```python
from build123d import *

# Parameters (mm, degrees)
BOSS_EXTRUDE1_DEPTH = 1.5
CUT_EXTRUDE6_DEPTH  = 11.5
CUT_EXTRUDE7_DEPTH  = 11.5


with BuildPart() as part:
    # 3DSketch1 → Boss-Extrude1 (new, along a direction that is not the sketch's normal)
    with BuildSketch(Plane(origin=(-11.663984258, 358.235252064, 0), x_dir=(0.8242948566390451, -0.5203008813923206, 0.22321510285101764), z_dir=(-0.26553281531955075, -0.007074831163105001, 0.964075863587761))):
        Polygon((0, 0), (489.889504132, 504.199636792), (815.132069395, 0), (238.511214526, -369.746400314), align=None)
    extrude(amount=BOSS_EXTRUDE1_DEPTH, dir=(0, 0, 1))

    # Sketch2 → Cut-Extrude6 (cut)
    with BuildSketch(Plane(origin=(-0.533410404, -0.014212136, 1.936664949), x_dir=(0.9641018224173596, -0.0019485492019291684, 0.26552566574162595), z_dir=(-0.26553281531954953, -0.007074831163105186, 0.9640758635877613))):
        with BuildLine():
            ThreePointArc((635.382584147, -65.776722047), (337.840777347, 133.826895304), (50.610501363, -80.349432548))
            Line((50.610501363, -80.349432548), (635.382584147, -65.776722047))
        make_face()
    extrude(amount=-CUT_EXTRUDE6_DEPTH, mode=Mode.SUBTRACT)

    # Sketch3 → Cut-Extrude7 (cut)
    with BuildSketch(Plane(origin=(-0.533410404, -0.014212136, 1.936664949), x_dir=(0.9641018224173596, -0.0019485492019291684, 0.26552566574162595), z_dir=(-0.26553281531954953, -0.007074831163105186, 0.9640758635877613))):
        Polygon((50.610501363, -80.349432548), (50.610501363, -106.198699681), (633.779172918, -106.198699681), (635.382584147, -65.776722047), (592.923417402, -33.337692785), (162.965228398, -33.337692785), align=None)
    extrude(amount=-CUT_EXTRUDE7_DEPTH, mode=Mode.SUBTRACT)


solid = part.part
```
Read the model definition and answer for the solid it produces. Units are mm, in the model's axes. Give positions to 0.01 mm unless a question says otherwise; leave off trailing zeros. Loops run counter-clockwise (first coordinate to the right, second up) from the corner with the lowest first, then second, coordinate; pieces in that order, holes last.
Item 1: The part is cut by section B-B (y = 260). Write down the section's boundary in (x, z).
Item 2: Find the intervals of material crossed by line 1 along Z through (x, y) = (594, 229.5); line 2 along Z through (x, y) = (146, 369.5), in increasing order.
Item 3: The mould has two halves that part along Z. Classify faces 1 (the flat face through (311.709, 444.842, 90.441)), 2 (the cylindrical face through (330.524, 133.233, 93.357)): released by +Z, released by -Z, zero draft, split by the parting line, or undercut.
Item 4: The part is cut by section A-A (y = 460). Write down the section's boundary in (x, z).
Item 5: Each of these flat-tipped pins is pushed along its axis until it touches: pin 1 Ø5 at (x, y) = (529, 71.5) entering from +Z; pin 2 Ø3 at (x, y) = (67, 339) entering from +Z. Where does it stop, or does it pass through?
Taken from the geometry:
1. outline: (-9.05, 0) - (651.56, 181.95) - (651.56, 183.45) - (-9.05, 1.5) - close
2. line 1: z = 165.87 to 167.37
2. line 2: z = 43.51 to 45.01
3. face 1: zero draft
3. face 2: split by the parting line
4. outline: (368.31, 105.4) - (646.23, 181.95) - (646.23, 183.45) - (368.31, 106.9) - close
5. pin 1: stops at z = 149
5. pin 2: stops at z = 23.44
